The model under review builds one solid part; all positions refer to its coordinate system, in mm. Face numbers are marked on the shaded views. A direction names the side the tool comes from. Give positions to 0.01 mm unless a question says otherwise; leave off trailing zeros. Write each loop counter-clockwise with the first axis right and the second up, starting at its lowest first coordinate (ties: lowest second). Pieces come first, ordered by that corner, then holes. Notation, with made-up numbers: M 6,67 L 18,67 A23 ccw 18,97 Z; hole C 73.5,-34.75 d8. An arc over 180 degrees is marked long. Write each question's results on one line, items separated by ' | '. Start each with the question number.
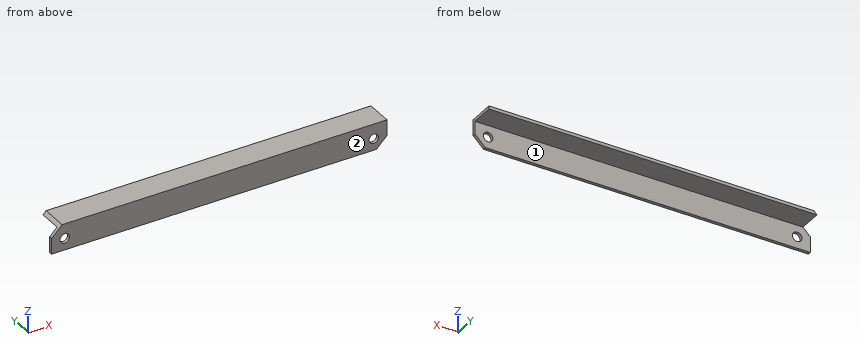
from build123d import *

# Parameters (mm, degrees)
F0_W     = 637
F0_H     = 50
F1_DEPTH = 6
F2_W     = 637
F2_H     = 6
F3_DEPTH = 44
F4_R     = 9
F5_DEPTH = 25
F7_DEPTH = 50


with BuildPart() as f1:
    # F0 (on Front) → F1 (new body)
    with BuildSketch(Plane.XZ):
        with Locations((318.5, 25)):
            Rectangle(F0_W, F0_H)
    extrude(amount=F1_DEPTH)

    # F2 (on face) → F3 (join)
    with BuildSketch(Plane(origin=(0, 0, 0), x_dir=(-1, 0, 0), z_dir=(0, 1, 0))):
        with Locations((-318.5, 47)):
            Rectangle(F2_W, F2_H)
    extrude(amount=F3_DEPTH)

    # F4 (on face) → F5 (cut)
    with BuildSketch(Plane.XZ.offset(6)):
        with Locations((25, 22)):
            Circle(F4_R)
        with Locations((612, 22)):
            Circle(F4_R)
    extrude(amount=-F5_DEPTH, mode=Mode.SUBTRACT)

    # F6 (on face) → F7 (cut)
    with BuildSketch(Plane.XZ.offset(6)):
        Polygon((637, 20), (617, 0), (637, 0), align=None)
        Polygon((0, 50), (0, 30), (20, 50), align=None)
    extrude(amount=-F7_DEPTH, mode=Mode.SUBTRACT)


solid = f1.part
(1) Machinability: for the marked faces 1 and 2, which of the approach directions +Z, -Z, +X, -X, +Y, -Y give a long, thin tool a straight path to every point of the face, cutting with its end or side? Answer none if there is none.
(2) Clearance check with a flat-ended pin moving along its axis: P1, Ø2, axis at x = 96.5, y = 3.5, coming from the -Z side. State where the tip first meets the part, or that it passes through.
(3) Wall thickness on L1, parallel to Z at x = 25, y = -3.15; L2, parallel to Y at x = 418.5, z = 37.5; L3, parallel to Z at x = 445, y = 29.5: over which ranges is each line inside the solid? List them lowest first.
(4) Add section A-A (x = 136.5). State the section outline as (y, z) points, then the cut area to 3 significant figures.
(5) Add section B-B (y = 22.5). State the section outline as (x, z) points, then the cut area to 3 significant figures.
Calculated:
1) face 1: -Z, +X, -X, +Y | face 2: +Z, -Z, +X, -X, -Y
2) P1: stops at z = 44
3) L1: z = 0 to 13, 31 to 50 | L2: y = -6 to 0 | L3: z = 44 to 50
4) outline: M -6,0 L 0,0 L 0,44 L 44,44 L 44,50 L -6,50 Z | area: 564 mm²
5) outline: M 14,44 L 637,44 L 637,50 L 20,50 Z | area: 3,720 mm²
